The model under review builds one solid part; all positions refer to its coordinate system, in mm. Round coordinates to 2 decimals unless told otherwise and drop trailing zeros. Write each loop counter-clockwise with the first axis right and the second up, starting at its lowest first coordinate (ties: lowest second). Pieces come first, ordered by that corner, then holes. Notation, with made-up numbers: (50, 40.5) -> (73, 40.5) arc R11 cw to (73, 55.5) -> close; hole circle Ø3 at (15.5, 57). An arc over 180 degrees is marked (long way). Answer as a JSON object with one key per item and string values. Group by question number.
1) We need section B-B, the plane x = -14.5. Write out the cut boundary in (y, z), then the cut area to 3 significant figures.
2) We need section A-A, the plane y = 12.5. Write out the cut boundary in (x, z).
3) Insertion check: pin 1 Ø4 at (x, y) = (-9, 8.5) entering from -Z; pin 2 Ø3 at (x, z) = (-52.11, 64.42) entering from -Y; pin 3 Ø12 at (y, z) = (2, -45) entering from -X; pin 4 Ø3 at (y, z) = (15, 39.5) entering from +X. Each pin has a flat end and moves straight along its axis. Give the tip position at first contact, or say it passes through.
4) We need section D-D, the plane z = 56.5. Write out the cut boundary in (x, y).
5) To check wall thickness, follow probe 1 along Y at (x, z) = (-36.5, -76); probe 2 along Z at (x, y) = (1.5, 3.25); probe 3 along Z at (x, y) = (19.5, 4). State the ranges of each line that lie inside material, in increasing order. Write a range as [from, to].
6) We need section C-C, the plane y = 2.5. Count the separate pieces of the cut face and the enclosed holes in it, then the cut area to 3 significant figures.
from build123d import *

# Parameters (mm, degrees)
BOSS_EXTRUDE1_DEPTH = 5
SKETCH2_R           = 2.2
CUT_EXTRUDE1_DEPTH  = 142.509716981
SKETCH3_R           = 1.1
SKETCH3_R_2         = 1.6
CUT_EXTRUDE3_DEPTH  = 142.509716981
SKETCH3_3_W         = 20
SKETCH3_3_H         = 4
SKETCH3_3_W_2       = 4
SKETCH3_3_H_2       = 25
BOSS_EXTRUDE2_DEPTH = 15
FILLET1_R           = 1


with BuildPart() as part:
    # Sketch1 → Boss-Extrude1 (new body)
    with BuildSketch(Plane(origin=(0, 0, 0), x_dir=(1, 0, 0), z_dir=(0, 1, 0))):
        with BuildLine():
            Line((97.353237465, -22.854915336), (22.854915336, -97.353237465))
            ThreePointArc((22.854915336, -97.353237465), (0, -100), (-22.854915336, -97.353237465))
            Line((-22.854915336, -97.353237465), (-97.353237465, -22.854915336))
            ThreePointArc((-97.353237465, -22.854915336), (-100, 0), (-97.353237465, 22.854915336))
            Line((-97.353237465, 22.854915336), (-22.854915336, 97.353237465))
            ThreePointArc((-22.854915336, 97.353237465), (0, 100), (22.854915336, 97.353237465))
            Line((22.854915336, 97.353237465), (97.353237465, 22.854915336))
            ThreePointArc((97.353237465, 22.854915336), (100, 0), (97.353237465, -22.854915336))
        make_face()
    extrude(amount=BOSS_EXTRUDE1_DEPTH)

    # Sketch2 → Cut-Extrude1 (cut, through all)
    with BuildSketch(Plane(origin=(0, 5, 0), x_dir=(1, 0, 0), z_dir=(0, 1, 0))):
        with Locations(Location((-40, -70, 0), (0, 0, 270))):
            Circle(SKETCH2_R)
        with Locations(Location((40, -70, 0), (0, 0, 270))):
            Circle(SKETCH2_R)
        with Locations(Location((40, 70, 0), (0, 0, 270))):
            Circle(SKETCH2_R)
        with Locations(Location((-40, 70, 0), (0, 0, 270))):
            Circle(SKETCH2_R)
        with Locations(Location((-70, 0, 0), (0, 0, 270))):
            Circle(SKETCH2_R)
        with Locations(Location((70, 0, 0), (0, 0, 270))):
            Circle(SKETCH2_R)
        with Locations(Location((7, -14, 0), (0, 0, 270))):
            Circle(SKETCH2_R)
        with Locations(Location((7, 14, 0), (0, 0, 90))):
            Circle(SKETCH2_R)
    extrude(amount=-CUT_EXTRUDE1_DEPTH, mode=Mode.SUBTRACT)

    # Sketch3 → Cut-Extrude3 (cut, through all)
    with BuildSketch(Plane(origin=(0, 5, 0), x_dir=(1, 0, 0), z_dir=(0, 1, 0))):
        with Locations(Location((-52.113769773, -64.417427766, 0), (0, 0, 270))):
            Circle(SKETCH3_R)
        with Locations(Location((-64.417427766, -52.113769773, 0), (0, 0, 270))):
            Circle(SKETCH3_R)
        with Locations(Location((64.417427766, -52.113769773, 0), (0, 0, 270))):
            Circle(SKETCH3_R)
        with Locations(Location((52.113769773, -64.417427766, 0), (0, 0, 270))):
            Circle(SKETCH3_R)
        with Locations(Location((64.417427766, 52.113769773, 0), (0, 0, 270))):
            Circle(SKETCH3_R)
        with Locations(Location((52.113769773, 64.417427766, 0), (0, 0, 270))):
            Circle(SKETCH3_R)
        with Locations(Location((-52.113769773, 64.417427766, 0), (0, 0, 270))):
            Circle(SKETCH3_R)
        with Locations(Location((-64.417427766, 52.113769773, 0), (0, 0, 270))):
            Circle(SKETCH3_R)
        with Locations(Location((19.00358005, -7.89, 0), (0, 0, 270))):
            Circle(SKETCH3_R_2)
        with Locations(Location((19.00358005, 7.89, 0), (0, 0, 270))):
            Circle(SKETCH3_R_2)
    extrude(amount=-CUT_EXTRUDE3_DEPTH, mode=Mode.SUBTRACT)

    # Sketch3_3 → Boss-Extrude2 (add)
    with BuildSketch(Plane(origin=(0, 5, 0), x_dir=(1, 0, 0), z_dir=(0, 1, 0))):
        with Locations((-12, -37.5)):
            Rectangle(SKETCH3_3_W, SKETCH3_3_H)
        with Locations((-32, 0)):
            Rectangle(SKETCH3_3_W_2, SKETCH3_3_H_2)
        with Locations((-12, 37.5)):
            Rectangle(SKETCH3_3_W, SKETCH3_3_H)
    extrude(amount=BOSS_EXTRUDE2_DEPTH)

    # Fillet1
    fillet1_edges = [part.edges().sort_by_distance(p)[0] for p in [
        (-12, 20, 35.5),
        (-2, 12.5, 35.5),
        (-22, 12.5, 35.5),
        (-30, 12.5, -12.5),
        (-30, 20, 0),
        (-30, 12.5, 12.5),
        (-22, 12.5, -35.5),
        (-2, 12.5, -35.5),
        (-12, 20, -35.5),
    ]]
    fillet(fillet1_edges, radius=FILLET1_R)


solid = part.part
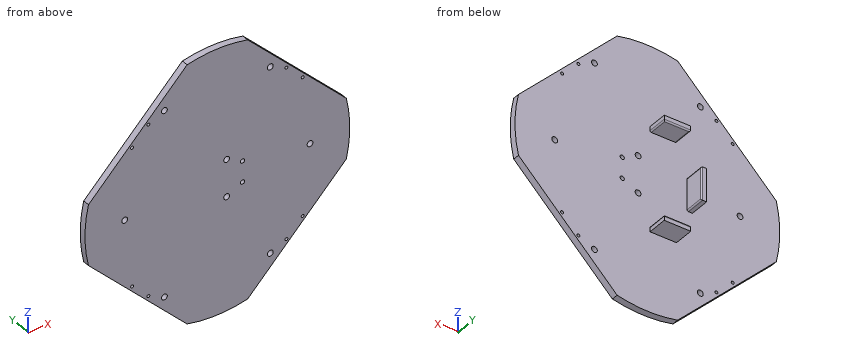
Here are the results:
{
 "1": {"outline": "(0, -98.94) -> (5, -98.94) -> (5, -39.5) -> (20, -39.5) -> (20, -36.5) arc R1 ccw to (19, -35.5) -> (5, -35.5) -> (5, 35.5) -> (19, 35.5) arc R1 ccw to (20, 36.5) -> (20, 39.5) -> (5, 39.5) -> (5, 98.94) -> (0, 98.94) -> close", "area": "1,110 mm^2"},
 "2": {"outline": "(-34, -12.5) -> (-31, -12.5) arc R1 ccw to (-30, -11.5) -> (-30, 11.5) arc R1 ccw to (-31, 12.5) -> (-34, 12.5) -> close; (-22, -39.5) -> (-2, -39.5) -> (-2, -36.5) arc R1 ccw to (-3, -35.5) -> (-21, -35.5) arc R1 ccw to (-22, -36.5) -> close; (-22, 36.5) arc R1 ccw to (-21, 35.5) -> (-3, 35.5) arc R1 ccw to (-2, 36.5) -> (-2, 39.5) -> (-22, 39.5) -> close"},
 "3": {"pin 1": "stops at z = -39.5", "pin 2": "stops at y = 0", "pin 3": "stops at x = -81.21", "pin 4": "stops at x = -2"},
 "4": {"outline": "(-63.71, 0) -> (63.71, 0) -> (63.71, 5) -> (-63.71, 5) -> close"},
 "5": {"probe 1": "y = [0, 5]", "probe 2": "z = [-99.99, 99.99]", "probe 3": "z = [-98.08, -9.41], [-6.37, 6.37], [9.41, 98.08]"},
 "6": {"separate pieces": "1", "enclosed holes": "18", "area": "27,000 mm^2"}
}
